Geometry: final body of the model. Coordinates: model frame, mm. A direction names the side the tool comes from. Round coordinates to 2 decimals unless told otherwise and drop trailing zeros. Loops run counter-clockwise (first coordinate to the right, second up) from the corner with the lowest first, then second, coordinate; pieces in that order, holes last. Notation, with made-up numbers: (62.5, 49) -> (120.5, 49) arc R23 ccw to (120.5, 86) -> close; hole circle Ø3 at (26.25, 75.25). An arc over 180 degrees is marked (long way). Answer in a Markdown table with one row per item.
```python
from build123d import *

# Parameters (mm, degrees)
SKETCH005_W  = 112.87
SKETCH005_H  = 87.5
PAD_DEPTH    = 2.2
SKETCH006_W  = 112.87
SKETCH006_H  = 87.5
PAD001_DEPTH = 2.2
SKETCH007_W  = 112.87
SKETCH007_H  = 87.5
SKETCH007_R  = 1.75
PAD002_DEPTH = 1.2
SKETCH008_W  = 112.87
SKETCH008_H  = 87.5
PAD003_DEPTH = 1.7
SKETCH010_W  = 112.87
SKETCH010_H  = 20
SKETCH010_R  = 2.2
PAD004_DEPTH = 2.2
FILLET_R     = 1


with BuildPart() as part:
    # Sketch005 → Pad (new body)
    with BuildSketch(Plane.XY):
        Rectangle(SKETCH005_W, SKETCH005_H)
        Polygon((-47.980514, 36.35), (-47.980514, 39.75), (-50.925, 41.45), (-53.869486, 39.75), (-53.869486, 36.35), (-50.925, 34.65), align=None, mode=Mode.SUBTRACT)
        Polygon((53.869486, 36.35), (53.869486, 39.75), (50.925, 41.45), (47.980514, 39.75), (47.980514, 36.35), (50.925, 34.65), align=None, mode=Mode.SUBTRACT)
        Polygon((53.869486, -36.35), (50.925, -34.65), (47.980514, -36.35), (47.980514, -39.75), (50.925, -41.45), (53.869486, -39.75), align=None, mode=Mode.SUBTRACT)
        Polygon((-47.980514, -39.75), (-47.980514, -36.35), (-50.925, -34.65), (-53.869486, -36.35), (-53.869486, -39.75), (-50.925, -41.45), align=None, mode=Mode.SUBTRACT)
    extrude(amount=PAD_DEPTH)

    # Sketch006 → Pad001 (join)
    with BuildSketch(Plane.XY.offset(2.2)):
        Rectangle(SKETCH006_W, SKETCH006_H)
        with BuildLine():
            Line((55.235, 33.85), (55.235, -33.85))
            Line((50.925, -33.85), (55.235, -33.85))
            ThreePointArc((50.925, -33.85), (47.955152, -35.080152), (46.725, -38.05))
            Line((46.725, -38.05), (46.725, -42.55))
            Line((46.725, -42.55), (-46.725, -42.55))
            Line((-46.725, -38.05), (-46.725, -42.55))
            ThreePointArc((-46.725, -38.05), (-47.955152, -35.080152), (-50.925, -33.85))
            Line((-50.925, -33.85), (-55.235, -33.85))
            Line((-55.235, -33.85), (-55.235, 33.85))
            Line((-55.235, 33.85), (-50.925, 33.85))
            ThreePointArc((-50.925, 33.85), (-47.955152, 35.080152), (-46.725, 38.05))
            Line((-46.725, 42.55), (-46.725, 38.05))
            Line((-46.725, 42.55), (46.725, 42.55))
            Line((46.725, 38.05), (46.725, 42.55))
            ThreePointArc((46.725, 38.05), (47.955152, 35.080152), (50.925, 33.85))
            Line((50.925, 33.85), (55.235, 33.85))
        make_face(mode=Mode.SUBTRACT)
        Polygon((-47.980514, 36.35), (-47.980514, 39.75), (-50.925, 41.45), (-53.869486, 39.75), (-53.869486, 36.35), (-50.925, 34.65), align=None, mode=Mode.SUBTRACT)
        Polygon((53.869486, 36.35), (53.869486, 39.75), (50.925, 41.45), (47.980514, 39.75), (47.980514, 36.35), (50.925, 34.65), align=None, mode=Mode.SUBTRACT)
        Polygon((53.869486, -36.35), (50.925, -34.65), (47.980514, -36.35), (47.980514, -39.75), (50.925, -41.45), (53.869486, -39.75), align=None, mode=Mode.SUBTRACT)
        Polygon((-47.980514, -39.75), (-47.980514, -36.35), (-50.925, -34.65), (-53.869486, -36.35), (-53.869486, -39.75), (-50.925, -41.45), align=None, mode=Mode.SUBTRACT)
    extrude(amount=PAD001_DEPTH)

    # Sketch007 → Pad002 (join)
    with BuildSketch(Plane.XY.offset(4.4)):
        Rectangle(SKETCH007_W, SKETCH007_H)
        with Locations((-50.925, 38.05)):
            Circle(SKETCH007_R, mode=Mode.SUBTRACT)
        with Locations((50.925, 38.05)):
            Circle(SKETCH007_R, mode=Mode.SUBTRACT)
        with Locations((50.925, -38.05)):
            Circle(SKETCH007_R, mode=Mode.SUBTRACT)
        with Locations((-50.925, -38.05)):
            Circle(SKETCH007_R, mode=Mode.SUBTRACT)
        with BuildLine():
            Line((55.235, 33.85), (55.235, -33.85))
            Line((50.925, -33.85), (55.235, -33.85))
            ThreePointArc((50.925, -33.85), (47.955152, -35.080152), (46.725, -38.05))
            Line((46.725, -38.05), (46.725, -42.55))
            Line((46.725, -42.55), (-46.725, -42.55))
            Line((-46.725, -38.05), (-46.725, -42.55))
            ThreePointArc((-46.725, -38.05), (-47.955152, -35.080152), (-50.925, -33.85))
            Line((-50.925, -33.85), (-55.235, -33.85))
            Line((-55.235, -33.85), (-55.235, 33.85))
            Line((-55.235, 33.85), (-50.925, 33.85))
            ThreePointArc((-50.925, 33.85), (-47.955152, 35.080152), (-46.725, 38.05))
            Line((-46.725, 42.55), (-46.725, 38.05))
            Line((-46.725, 42.55), (46.725, 42.55))
            Line((46.725, 38.05), (46.725, 42.55))
            ThreePointArc((46.725, 38.05), (47.955152, 35.080152), (50.925, 33.85))
            Line((50.925, 33.85), (55.235, 33.85))
        make_face(mode=Mode.SUBTRACT)
    extrude(amount=PAD002_DEPTH)

    # Sketch008 → Pad003 (join)
    with BuildSketch(Plane.XY.offset(5.6)):
        Rectangle(SKETCH008_W, SKETCH008_H)
        Polygon((55.235, 33.85), (55.235, -33.85), (55.235, -42.55), (46.725, -42.55), (-46.725, -42.55), (-55.235, -42.55), (-55.235, -33.85), (-55.235, 33.85), (-55.235, 42.55), (-46.725, 42.55), (46.725, 42.55), (55.235, 42.55), align=None, mode=Mode.SUBTRACT)
    extrude(amount=PAD003_DEPTH)

    # Sketch010 → Pad004 (join)
    with BuildSketch(Plane.XY):
        with Locations((0, 53.75)):
            Rectangle(SKETCH010_W, SKETCH010_H)
        with Locations((-41.435, 53.75)):
            Circle(SKETCH010_R, mode=Mode.SUBTRACT)
        with Locations((41.435, 53.75)):
            Circle(SKETCH010_R, mode=Mode.SUBTRACT)
    extrude(amount=PAD004_DEPTH)

    # Fillet
    fillet_edges = [part.edges().sort_by_distance(p)[0] for p in [
        (-56.435, 10, 0),
        (46.725, 40.3, 2.2),
        (0, 42.55, 2.2),
        (-46.725, 40.3, 2.2),
        (-47.955152, 35.080152, 2.2),
        (-53.08, 33.85, 2.2),
        (-55.235, 0, 2.2),
        (-53.08, -33.85, 2.2),
        (-47.955152, -35.080152, 2.2),
        (-46.725, -40.3, 2.2),
        (0, -42.55, 2.2),
        (46.725, -40.3, 2.2),
        (47.955152, -35.080152, 2.2),
        (53.08, -33.85, 2.2),
        (55.235, 0, 2.2),
        (53.08, 33.85, 2.2),
        (47.955152, 35.080152, 2.2),
        (0, -43.75, 0),
        (56.435, 10, 0),
        (56.435, -43.75, 3.65),
        (56.435, 43.75, 4.75),
        (56.435, 53.75, 2.2),
        (56.435, 63.75, 1.1),
        (-56.435, 63.75, 1.1),
        (-56.435, 53.75, 2.2),
        (0, 63.75, 2.2),
        (-56.435, 43.75, 4.75),
        (-56.435, -43.75, 3.65),
    ]]
    fillet(fillet_edges, radius=FILLET_R)


solid = part.part
```
Item 1: Cut plane C-C (y = 12). Output: boundary loops of the cut face in (x, z) (3 decimals).
Answer:
| item | result |
|---|---|
| outline | (-56.435, 1) arc R1 ccw to (-55.435, 0) -> (55.435, 0) arc R1 ccw to (56.435, 1) -> (56.435, 7.3) -> (55.235, 7.3) -> (55.235, 3.2) arc R1 cw to (54.235, 2.2) -> (-54.235, 2.2) arc R1 cw to (-55.235, 3.2) -> (-55.235, 7.3) -> (-56.435, 7.3) -> close |
Item 2: Cut plane D-D (x = 6). Output: boundary loops of the cut face in (y, z).
Answer:
| item | result |
|---|---|
| outline | (-43.75, 1) arc R1 ccw to (-42.75, 0) -> (63.75, 0) -> (63.75, 1.2) arc R1 ccw to (62.75, 2.2) -> (43.75, 2.2) -> (43.75, 7.3) -> (42.55, 7.3) -> (42.55, 3.2) arc R1 cw to (41.55, 2.2) -> (-41.55, 2.2) arc R1 cw to (-42.55, 3.2) -> (-42.55, 7.3) -> (-43.75, 7.3) -> close |
Item 3: Cut plane A-A (y = 53.75). Output: boundary loops of the cut face in (x, z) (3 decimals).
Answer:
| item | result |
|---|---|
| outline | (-56.435, 1) arc R1 ccw to (-55.435, 0) -> (-43.635, 0) -> (-43.635, 2.2) -> (-55.435, 2.2) arc R1 ccw to (-56.435, 1.2) -> close; (-39.235, 0) -> (39.235, 0) -> (39.235, 2.2) -> (-39.235, 2.2) -> close; (43.635, 0) -> (55.435, 0) arc R1 ccw to (56.435, 1) -> (56.435, 1.2) arc R1 ccw to (55.435, 2.2) -> (43.635, 2.2) -> close |
Item 4: Pin query (flat end, axial travel): pin 1 Ø2.5 at (x, y) = (41.435, 53.75) entering from +Z (3 decimals); pin 2 Ø1 at (x, z) = (-14, 4.5) entering from +Y; pin 3 Ø8 at (x, y) = (19, -1) entering from +Z; pin 4 Ø5.5 at (x, y) = (50.925, 38.05) entering from +Z. Return the tip coordinate at first contact, or that it passes through.
Answer:
| item | result |
|---|---|
| pin 1 | passes through |
| pin 2 | stops at y = 43.75 |
| pin 3 | stops at z = 2.2 |
| pin 4 | stops at z = 5.6 |
Item 5: Draft query along Y for faces 4 (the face through (-1, 11, 0)), 5 (the face through (53, -33.85, 4)). Return one class per face: pulls with the +Y half, pulls with the -Y half, needs draft (parallel to the pull), parting line crosses it, or undercut.
Answer:
| item | result |
|---|---|
| face 4 | needs draft |
| face 5 | undercut |
Item 6: Cut plane B-B (x = 41). Output: boundary loops of the cut face in (y, z).
Answer:
| item | result |
|---|---|
| outline | (-43.75, 1) arc R1 ccw to (-42.75, 0) -> (51.59, 0) -> (51.59, 2.2) -> (43.75, 2.2) -> (43.75, 7.3) -> (42.55, 7.3) -> (42.55, 3.2) arc R1 cw to (41.55, 2.2) -> (-41.55, 2.2) arc R1 cw to (-42.55, 3.2) -> (-42.55, 7.3) -> (-43.75, 7.3) -> close; (55.91, 0) -> (63.75, 0) -> (63.75, 1.2) arc R1 ccw to (62.75, 2.2) -> (55.91, 2.2) -> close |
Item 7: Reachability of faces 1 (the face through (53, -38, 5.6)), 2 (the face through (-52.4, 40.6, 2.2)), 3 (the face through (-56.435, -2, 4)) from +Z, -Z, +X, -X, +Y, -Y: full face, straight path, thin tool, end or side. Return the list, or none.
Answer:
| item | result |
|---|---|
| face 1 | +Z |
| face 2 | -Z |
| face 3 | +Z, -Z, -X, +Y, -Y |
Item 8: Line query: probe 1 along X at (y, z) = (4.5, 3.75) (3 decimals); probe 2 along Y at (x, z) = (-48.5, 7); probe 3 along Z at (x, y) = (-25, -29). Output: solid intervals per line, ascending. Write a range as [from, to].
Answer:
| item | result |
|---|---|
| probe 1 | x = [-56.435, -55.235], [55.235, 56.435] |
| probe 2 | y = [-43.75, -42.55], [42.55, 43.75] |
| probe 3 | z = [0, 2.2] |
